Design review of the part shown in the three views and the two pictorial views. Dimensions are in mm from the part's minimum x, y and z. A direction names the side the tool comes from. Round coordinates to 2 decimals unless told otherwise and drop trailing zeros. Order: outer loops, then holes, each group sorted by start corner. A loop starts at its lowest first (then second) coordinate and runs counter-clockwise, first axis right, second up.
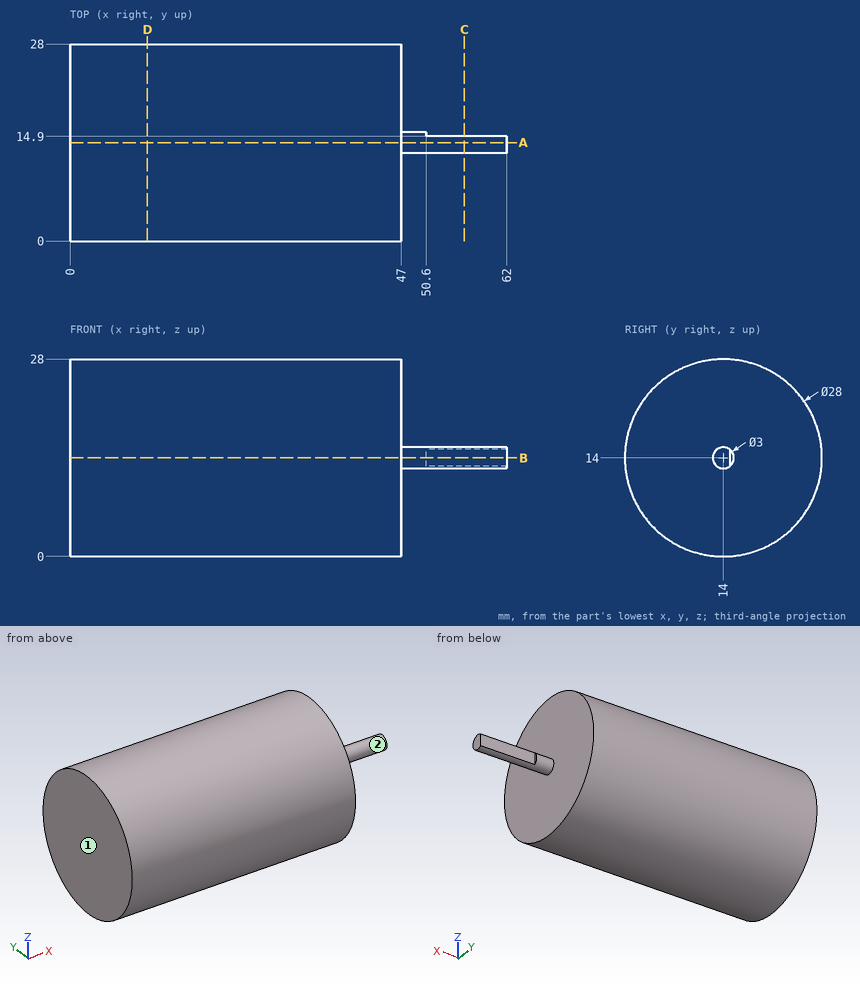
(1) Wall thickness on L1, parallel to X at y = 12, z = 19.25; L2, parallel to Z at x = 44.5, y = 13.75; L3, parallel to Z at x = 10, y = 2: over which ranges is each line inside the solid? List them lowest first.
(2) Add section D-D on x = 11. Give the boundary of the cut face in (y, z).
(3) Tool access review of the marked faces 1 and 2: name each direction out of +Z, -Z, +X, -X, +Y, -Y from which nothing blocks a thin tool from reaching the whole face with its end or side.
(4) Add section A-A on y = 14. Give the boundary of the cut face in (x, z).
(5) Add section B-B on z = 14. Give the boundary of the cut face in (x, y).
(6) Add section C-C on x = 56. Give the boundary of the cut face in (y, z), plus the area to 3 significant figures.
(7) Clearance check with flat-ended pins moving along their axes: P1, Ø3, axis at x = 29, z = 4.5, coming from the +Y side; P2, Ø4, axis at x = 41.5, z = 4.5, coming from the +Y side; P3, Ø3, axis at x = 28, y = 3, coming from the +Z side. State where each tip first meets the part, or that it passes through.
Here are the results:
1. L1: x = 0 to 47
1. L2: z = 0 to 28
1. L3: z = 6.79 to 21.21
2. outline: circle Ø28 at (14, 14)
3. face 1: +Z, -Z, -X, +Y, -Y
3. face 2: +X
4. outline: (0, 0) - (47, 0) - (47, 12.5) - (62, 12.5) - (62, 15.5) - (47, 15.5) - (47, 28) - (0, 28) - close
5. outline: (0, 0) - (47, 0) - (47, 12.5) - (62, 12.5) - (62, 14.9) - (50.6, 14.9) - (50.6, 15.5) - (47, 15.5) - (47, 28) - (0, 28) - close
6. outline: (14.9, 12.8) - (14.9, 15.2) arc R1.5 ccw (long way) to start
6. area: 6.06 mm2
7. P1: stops at y = 25.49
7. P2: stops at y = 25.82
7. P3: stops at z = 24.28
